```python
from build123d import *

# Parameters (mm, degrees)
CROQUIS1_R              = 4
SALIENTE_EXTRUIR1_DEPTH = 52
CROQUIS2_R              = 5
SALIENTE_EXTRUIR2_DEPTH = 5
CROQUIS3_R              = 4
CROQUIS3_R_2            = 3
CORTAR_EXTRUIR1_DEPTH   = 22
CROQUIS5_R              = 1.25
CORTAR_EXTRUIR2_DEPTH   = 54.009433123
CHAFL_N1_SIZE           = 0.5


# Read off the part's stored shape, not the designer's step: M8 Roscas Standard Taladro1
with BuildPart() as part:
    # Croquis1 → Saliente-Extruir1 (new, symmetric)
    with BuildSketch(Plane.XY):
        with Locations(Location((0, 0, 0), (0, 0, 180))):
            Circle(CROQUIS1_R)
    extrude(amount=SALIENTE_EXTRUIR1_DEPTH, both=True)

    # Croquis2 → Saliente-Extruir2 (add)
    with BuildSketch(Plane.XY.offset(-28.5)):
        Circle(CROQUIS2_R)
    extrude(amount=SALIENTE_EXTRUIR2_DEPTH)

    # Croquis3 → Cortar-Extruir1 (cut)
    with BuildSketch(Plane.XY.offset(52)):
        with Locations(Location((0, 0, 0), (0, 0, 180))):
            Circle(CROQUIS3_R)
        Circle(CROQUIS3_R_2, mode=Mode.SUBTRACT)
    extrude(amount=-CORTAR_EXTRUIR1_DEPTH, mode=Mode.SUBTRACT)

    # M8 Roscas Standard Taladro1 outline → M8 Roscas Standard Taladro1 (revolve, cut)
    with BuildSketch(Plane.XZ):
        Polygon((4, 30), (3.3095, 30), (4, 29.3095), align=None)
    revolve(axis=Axis((0, 0, 0), (0, 0, 1)), mode=Mode.SUBTRACT)

    # Croquis5 → Cortar-Extruir2 (cut, through all)
    with BuildSketch(Plane(origin=(0, 4, 0), x_dir=(1, 0, 0), z_dir=(0, 1, 0))):
        with Locations(Location((0, 41.5, 0), (0, 0, 270))):
            Circle(CROQUIS5_R)
    extrude(amount=-CORTAR_EXTRUIR2_DEPTH, mode=Mode.SUBTRACT)

    # Chaflán1
    chafl_n1_edges = [part.edges().sort_by_distance(p)[0] for p in [
        (-3, 0, 52),
        (4, 0, -52),
    ]]
    chamfer(chafl_n1_edges, length=CHAFL_N1_SIZE)


solid = part.part
```
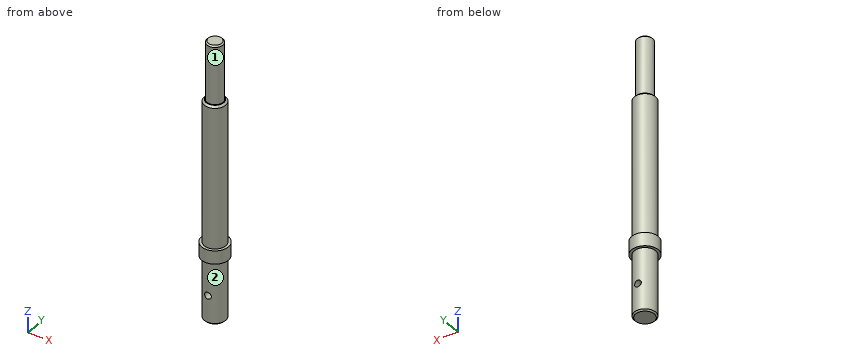
Here's how the part is built. I have some questions about the finished solid (model axes, mm). Face numbers are marked on the shaded views. A direction names the side the tool comes from. Round coordinates to 2 decimals unless told otherwise and drop trailing zeros. Loops run counter-clockwise (first coordinate to the right, second up) from the corner with the lowest first, then second, coordinate; pieces in that order, holes last.
1. If I drill on probe 1 along Z at (x, y) = (0, -1.5); probe 2 along X at (y, z) = (0.25, -41.5); probe 3 along Y at (x, z) = (0.25, -40), over which ranges is the centre line in solid material (lowest first)?
Answers:
probe 1: z = -52 to -42.75, -40.25 to 52
probe 2: x = -3.99 to -1.25, 1.25 to 3.99
probe 3: y = -3.99 to 3.99
2. Will these pins go through, and if not, where does the flat tip stop? pin 1 (1 mm diameter, centred on x = -4, y = -1.5, fed in from -Z); pin 2 (5 mm diameter, centred on x = 2, z = -10.5, fed in from +Y); pin 3 (4 mm diameter, centred on y = 0.5, z = -8.5, fed in from -X).
Answers:
pin 1: stops at z = -51.73
pin 2: stops at y = 4
pin 3: stops at x = -4
3. For the marked faces 1 and 2, which set-ups out of +Z, -Z, +X, -X, +Y, -Y let a thin tool reach every point of the face, with its end or its side?
Answers:
face 1: +Z
face 2: -Z
4. Suppose I cut it at C-C, the plane z = -41.5. Please give me the cut outline in (x, y).
Answers:
outline: (-1.25, -3.8) - (-1.25, 3.8) arc R4 ccw to start; (1.25, -3.8) arc R4 ccw to (1.25, 3.8) - close
5. Suppose I cut it at A-A, the plane x = 0. Please give me the cut outline in (y, z).
Answers:
outline: (-5, -28.5) - (-4, -28.5) - (-4, -40.25) - (4, -40.25) - (4, -28.5) - (5, -28.5) - (5, -23.5) - (4, -23.5) - (4, 29.31) - (3.31, 30) - (3, 30) - (3, 51.5) - (2.5, 52) - (-2.5, 52) - (-3, 51.5) - (-3, 30) - (-3.31, 30) - (-4, 29.31) - (-4, -23.5) - (-5, -23.5) - close; (-4, -51.5) - (-3.5, -52) - (3.5, -52) - (4, -51.5) - (4, -42.75) - (-4, -42.75) - close
6. Suppose I cut it at B-B, the plane y = 0. Please give me the cut outline in (x, z).
Answers:
outline: (-5, -28.5) - (-4, -28.5) - (-4, -51.5) - (-3.5, -52) - (3.5, -52) - (4, -51.5) - (4, -28.5) - (5, -28.5) - (5, -23.5) - (4, -23.5) - (4, 29.31) - (3.31, 30) - (3, 30) - (3, 51.5) - (2.5, 52) - (-2.5, 52) - (-3, 51.5) - (-3, 30) - (-3.31, 30) - (-4, 29.31) - (-4, -23.5) - (-5, -23.5) - close; hole circle Ø2.5 at (0, -41.5)
